Geometry: final body of the model. Coordinates: model frame, mm. A direction names the side the tool comes from. Coordinates: 2 decimals unless noted, no trailing zeros. Write each loop counter-clockwise with the first axis right and the second up, starting at its lowest first coordinate (ties: lowest second). Pieces come first, ordered by that corner, then holes. Notation, with made-up numbers: (-24, 11.5) - (13, 11.5) arc R28 cw to (13, 47.5) - close; hole circle Ø4 at (-18.75, -33.5). An arc over 180 degrees is marked (long way). Answer as a JSON object with one key per item and string values. Group by question number.
Item 1: First-contact query: pin 1 Ø1.5 at (y, z) = (0.5, 8) entering from +X; pin 2 Ø3.5 at (x, y) = (0, 10) entering from -Z; pin 3 Ø6 at (x, z) = (10, 5) entering from -Y; pin 4 Ø2 at (x, z) = (6, 7.5) entering from -Y. Flat tips, straight axial feed; report the tip coordinate or a pass-through.
Item 2: Mould query, pull axis Y, two halves, no side actions, for faces 3 (the cylindrical face through (-7.46, -5.5, 8.18)), 4 (the cylindrical face through (11.923, 3.755, 8.071)), 5 (the flat face through (0, 0, 12)). Classes: pulls with the +Y half, pulls with the -Y half, needs draft (parallel to the pull), parting line crosses it, or undercut.
Item 3: Section C-C on y = 0. Return loops of the section in (x, z).
Item 4: Section B-B on x = 0. Return loops of the section in (y, z), and give its area (3 significant figures).
Item 5: Section A-A on y = 10. Return loops of the section in (x, z).
Item 6: Line query: line 1 along Y through (x, z) = (0, 6); line 2 along Z through (x, y) = (10.5, 0.5); line 3 along Y through (x, z) = (9.75, 6). Output: solid intervals per line, ascending. Write a range as from..to.
Item 7: Set-up query: faces 1 (the flat face through (3, -5.4, 4.25)), 2 (the cylindrical face through (8.38, -6.27, 8.18)). Return all of +Z, -Z, +X, -X, +Y, -Y with unobstructed straight access to the full face (end or side cutting, diameter ignored); none if empty.
Item 8: Section D-D on z = 5.5. Return loops of the section in (x, y), and give its area (3 significant figures).
```python
from build123d import *

# Parameters (mm, degrees)
SKETCH_1_R          = 12.5
EXTRUDE_1_DEPTH     = 12
SKETCH_2_R          = 1.3
CUT_EXTRUDE_1_DEPTH = 22.365860619
SKETCH_3_R          = 12.5
SKETCH_3_R_2        = 5
CUT_EXTRUDE_2_DEPTH = 4.25
EXTRUDE_START       = 1
SKETCH_4_R          = 6
SKETCH_4_R_2        = 5
EXTRUDE_2_DEPTH     = 1


with BuildPart() as part:
    # ｽｹｯﾁ1 → ﾎﾞｽ - 押し出し1 (new body)
    with BuildSketch(Plane.XY):
        Circle(SKETCH_1_R)
    extrude(amount=EXTRUDE_1_DEPTH)

    # ｽｹｯﾁ2 → ｶｯﾄ - 押し出し1 (cut, through all)
    with BuildSketch(Plane.XY.offset(12)):
        with Locations((0, 10)):
            Circle(SKETCH_2_R)
        with Locations((8.660254038, -5)):
            Circle(SKETCH_2_R)
        with Locations((-8.660254038, -5)):
            Circle(SKETCH_2_R)
    extrude(amount=-CUT_EXTRUDE_1_DEPTH, mode=Mode.SUBTRACT)

    # ｽｹｯﾁ3 → ｶｯﾄ - 押し出し2 (cut)
    with BuildSketch(Plane(origin=(0, 0, 0), x_dir=(-1, 0, 0), z_dir=(0, 0, -1))):
        Circle(SKETCH_3_R)
        Circle(SKETCH_3_R_2, mode=Mode.SUBTRACT)
    extrude(amount=-CUT_EXTRUDE_2_DEPTH, mode=Mode.SUBTRACT)

    # ｽｹｯﾁ4 → ﾎﾞｽ - 押し出し2 (add)
    with BuildSketch(Plane(origin=(0, 0, 4.25), x_dir=(-1, 0, 0), z_dir=(0, 0, -1)).offset(EXTRUDE_START)):
        Circle(SKETCH_4_R)
        Circle(SKETCH_4_R_2, mode=Mode.SUBTRACT)
    extrude(amount=-EXTRUDE_2_DEPTH)


solid = part.part
```
Checks:
{
 "1": {"pin 1": "x = 12.5", "pin 2": "z = 4.25", "pin 3": "y = -10.36", "pin 4": "y = -11.46"},
 "2": {"face 3": "undercut", "face 4": "parting line crosses it", "face 5": "needs draft"},
 "3": {"outline": "(-12.5, 4.25) - (-6, 4.25) - (-6, 3.25) - (-5, 3.25) - (-5, 0) - (5, 0) - (5, 3.25) - (6, 3.25) - (6, 4.25) - (12.5, 4.25) - (12.5, 12) - (-12.5, 12) - close"},
 "4": {"outline": "(-12.5, 4.25) - (-6, 4.25) - (-6, 3.25) - (-5, 3.25) - (-5, 0) - (5, 0) - (5, 3.25) - (6, 3.25) - (6, 4.25) - (8.7, 4.25) - (8.7, 12) - (-12.5, 12) - close; (11.3, 4.25) - (12.5, 4.25) - (12.5, 12) - (11.3, 12) - close", "area": "218 mm^2"},
 "5": {"outline": "(-7.5, 4.25) - (-1.3, 4.25) - (-1.3, 12) - (-7.5, 12) - close; (1.3, 4.25) - (7.5, 4.25) - (7.5, 12) - (1.3, 12) - close"},
 "6": {"line 1": "-12.5..8.7, 11.3..12.5", "line 2": "4.25..12", "line 3": "-7.82..-5.71, -4.29..7.82"},
 "7": {"face 1": "-Z", "face 2": "+Z, -Z"},
 "8": {"outline": "circle Ø25 at (0, 0); hole circle Ø2.6 at (-8.66, -5); hole circle Ø2.6 at (0, 10); hole circle Ø2.6 at (8.66, -5)", "area": "475 mm^2"}
}
